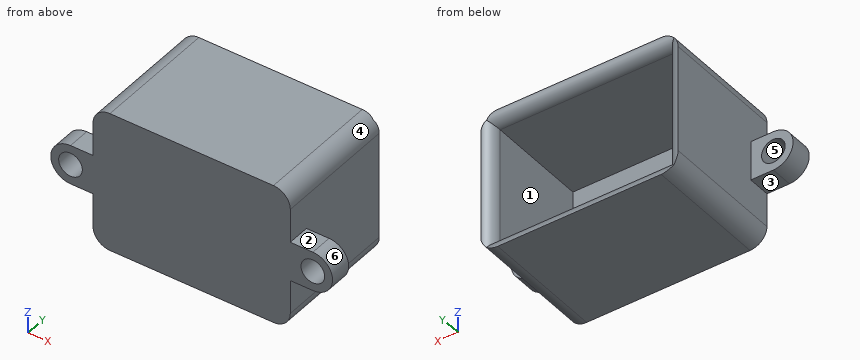
from build123d import *

# Parameters (mm, degrees)
SKETCH2_W           = 35
SKETCH2_H           = 25
SKETCH2_W_2         = 31
SKETCH2_H_2         = 21
BOSS_EXTRUDE1_DEPTH = 20
SKETCH3_W           = 35
SKETCH3_H           = 25
BOSS_EXTRUDE2_DEPTH = 2
SKETCH4_R           = 2.1
BOSS_EXTRUDE3_DEPTH = 4
FILLET1_R           = 3
FILLET2_R           = 2


with BuildPart() as part:
    # Sketch2 → Boss-Extrude1 (new body)
    with BuildSketch(Plane(origin=(0, 0, 0), x_dir=(1, 0, 0), z_dir=(0, 1, 0))):
        Rectangle(SKETCH2_W, SKETCH2_H)
        Rectangle(SKETCH2_W_2, SKETCH2_H_2, mode=Mode.SUBTRACT)
    extrude(amount=BOSS_EXTRUDE1_DEPTH)

    # Sketch3 → Boss-Extrude2 (add)
    with BuildSketch(Plane.XZ):
        Rectangle(SKETCH3_W, SKETCH3_H)
    extrude(amount=BOSS_EXTRUDE2_DEPTH)

    # Sketch4 → Boss-Extrude3 (add)
    # profile 1 of 2: a face of its own
    with BuildSketch(Plane.XZ.offset(2)):
        with BuildLine():
            Line((-21.5, 3.5), (-17.5, 3.5))
            Line((-17.5, 3.5), (-17.5, -3.5))
            Line((-17.5, -3.5), (-21.5, -3.5))
            ThreePointArc((-21.5, -3.5), (-25, 0), (-21.5, 3.5))
        make_face()
        with Locations(Location((-21.5, 0, 0), (0, 0, 270))):
            Circle(SKETCH4_R, mode=Mode.SUBTRACT)
    # profile 2 of 2: a face of its own
    with BuildSketch(Plane.XZ.offset(2)):
        with BuildLine():
            Line((17.5, 3.5), (17.5, -3.5))
            Line((17.5, -3.5), (21.5, -3.5))
            ThreePointArc((21.5, -3.5), (25, 0), (21.5, 3.5))
            Line((21.5, 3.5), (17.5, 3.5))
        make_face()
        with Locations(Location((21.5, 0, 0), (0, 0, 90))):
            Circle(SKETCH4_R, mode=Mode.SUBTRACT)
    extrude(amount=-BOSS_EXTRUDE3_DEPTH)

    # Fillet1
    fillet1_edges = [part.edges().sort_by_distance(p)[0] for p in [
        (17.5, 9, 12.5),
        (-17.5, 9, 12.5),
        (-17.5, 9, -12.5),
        (17.5, 9, -12.5),
    ]]
    fillet(fillet1_edges, radius=FILLET1_R)

    # Fillet2
    # the kernel refuses this fillet: 2 mm, written as the material it takes off along each edge
    with BuildSketch(Plane(origin=(15.5, 20, -10.5), x_dir=(1, 0, 0), z_dir=(0, 0, 1)), Plane(origin=(-15.5, 20, 10.5), x_dir=(-1, 0, 0), z_dir=(0, 0, -1))) as fillet2_piece_1:
        with BuildLine():
            CenterArc((FILLET2_R, -FILLET2_R), FILLET2_R, 90, 90)
            Line((0, -FILLET2_R), (-FILLET2_R * 0.02, -FILLET2_R))
            Line((-FILLET2_R * 0.02, -FILLET2_R), (-FILLET2_R * 0.02, FILLET2_R * 0.02))
            Line((-FILLET2_R * 0.02, FILLET2_R * 0.02), (FILLET2_R, FILLET2_R * 0.02))
            Line((FILLET2_R, FILLET2_R * 0.02), (FILLET2_R, 0))
        make_face()
    extrude(amount=21, mode=Mode.SUBTRACT)
    with BuildSketch(Plane(origin=(-15.5, 20, -10.5), x_dir=(0, 0, -1), z_dir=(1, 0, 0)), Plane(origin=(15.5, 20, 10.5), x_dir=(0, 0, 1), z_dir=(-1, 0, 0))) as fillet2_piece_2:
        with BuildLine():
            CenterArc((FILLET2_R, -FILLET2_R), FILLET2_R, 90, 90)
            Line((0, -FILLET2_R), (-FILLET2_R * 0.02, -FILLET2_R))
            Line((-FILLET2_R * 0.02, -FILLET2_R), (-FILLET2_R * 0.02, FILLET2_R * 0.02))
            Line((-FILLET2_R * 0.02, FILLET2_R * 0.02), (FILLET2_R, FILLET2_R * 0.02))
            Line((FILLET2_R, FILLET2_R * 0.02), (FILLET2_R, 0))
        make_face()
    extrude(amount=31, mode=Mode.SUBTRACT)
    with BuildSketch(Plane(origin=(15.5, 20, -15.5), x_dir=(1, 0, 0), z_dir=(0, 0, 1))) as fillet2_piece_3a_section:
        with BuildLine():
            CenterArc((FILLET2_R, -FILLET2_R), FILLET2_R, 90, 90)
            Line((0, -FILLET2_R), (-FILLET2_R * 0.02, -FILLET2_R))
            Line((-FILLET2_R * 0.02, -FILLET2_R), (-FILLET2_R * 0.02, FILLET2_R * 0.02))
            Line((-FILLET2_R * 0.02, FILLET2_R * 0.02), (FILLET2_R, FILLET2_R * 0.02))
            Line((FILLET2_R, FILLET2_R * 0.02), (FILLET2_R, 0))
        make_face()
    fillet2_piece_3a = extrude(amount=26, mode=Mode.PRIVATE)
    fillet2_piece_3a = split(fillet2_piece_3a, bisect_by=Plane(origin=(15.952790229, 19.547209771, -10.5), z_dir=(0, 0, -1)), keep=Keep.TOP, mode=Mode.PRIVATE)
    with BuildSketch(Plane(origin=(-15.5, 20, -10.5), x_dir=(0, 0, -1), z_dir=(1, 0, 0))) as fillet2_piece_3b_section:
        with BuildLine():
            CenterArc((FILLET2_R, -FILLET2_R), FILLET2_R, 90, 90)
            Line((0, -FILLET2_R), (-FILLET2_R * 0.02, -FILLET2_R))
            Line((-FILLET2_R * 0.02, -FILLET2_R), (-FILLET2_R * 0.02, FILLET2_R * 0.02))
            Line((-FILLET2_R * 0.02, FILLET2_R * 0.02), (FILLET2_R, FILLET2_R * 0.02))
            Line((FILLET2_R, FILLET2_R * 0.02), (FILLET2_R, 0))
        make_face()
    fillet2_piece_3b = extrude(amount=36, mode=Mode.PRIVATE)
    fillet2_piece_3b = split(fillet2_piece_3b, bisect_by=Plane(origin=(15.5, 19.547209771, -10.952790229), z_dir=(1, 0, 0)), keep=Keep.TOP, mode=Mode.PRIVATE)
    fillet2_piece_3 = fillet2_piece_3a & fillet2_piece_3b
    add(fillet2_piece_3, mode=Mode.SUBTRACT)
    with BuildSketch(Plane(origin=(20.5, 20, 10.5), x_dir=(0, 0, 1), z_dir=(-1, 0, 0))) as fillet2_piece_4a_section:
        with BuildLine():
            CenterArc((FILLET2_R, -FILLET2_R), FILLET2_R, 90, 90)
            Line((0, -FILLET2_R), (-FILLET2_R * 0.02, -FILLET2_R))
            Line((-FILLET2_R * 0.02, -FILLET2_R), (-FILLET2_R * 0.02, FILLET2_R * 0.02))
            Line((-FILLET2_R * 0.02, FILLET2_R * 0.02), (FILLET2_R, FILLET2_R * 0.02))
            Line((FILLET2_R, FILLET2_R * 0.02), (FILLET2_R, 0))
        make_face()
    fillet2_piece_4a = extrude(amount=36, mode=Mode.PRIVATE)
    fillet2_piece_4a = split(fillet2_piece_4a, bisect_by=Plane(origin=(15.5, 19.547209771, 10.952790229), z_dir=(1, 0, 0)), keep=Keep.TOP, mode=Mode.PRIVATE)
    with BuildSketch(Plane(origin=(15.5, 20, -10.5), x_dir=(1, 0, 0), z_dir=(0, 0, 1))) as fillet2_piece_4b_section:
        with BuildLine():
            CenterArc((FILLET2_R, -FILLET2_R), FILLET2_R, 90, 90)
            Line((0, -FILLET2_R), (-FILLET2_R * 0.02, -FILLET2_R))
            Line((-FILLET2_R * 0.02, -FILLET2_R), (-FILLET2_R * 0.02, FILLET2_R * 0.02))
            Line((-FILLET2_R * 0.02, FILLET2_R * 0.02), (FILLET2_R, FILLET2_R * 0.02))
            Line((FILLET2_R, FILLET2_R * 0.02), (FILLET2_R, 0))
        make_face()
    fillet2_piece_4b = extrude(amount=26, mode=Mode.PRIVATE)
    fillet2_piece_4b = split(fillet2_piece_4b, bisect_by=Plane(origin=(15.952790229, 19.547209771, 10.5), z_dir=(0, 0, 1)), keep=Keep.TOP, mode=Mode.PRIVATE)
    fillet2_piece_4 = fillet2_piece_4a & fillet2_piece_4b
    add(fillet2_piece_4, mode=Mode.SUBTRACT)
    with BuildSketch(Plane(origin=(-15.5, 20, 10.5), x_dir=(-1, 0, 0), z_dir=(0, 0, -1))) as fillet2_piece_5a_section:
        with BuildLine():
            CenterArc((FILLET2_R, -FILLET2_R), FILLET2_R, 90, 90)
            Line((0, -FILLET2_R), (-FILLET2_R * 0.02, -FILLET2_R))
            Line((-FILLET2_R * 0.02, -FILLET2_R), (-FILLET2_R * 0.02, FILLET2_R * 0.02))
            Line((-FILLET2_R * 0.02, FILLET2_R * 0.02), (FILLET2_R, FILLET2_R * 0.02))
            Line((FILLET2_R, FILLET2_R * 0.02), (FILLET2_R, 0))
        make_face()
    fillet2_piece_5a = extrude(amount=26, mode=Mode.PRIVATE)
    fillet2_piece_5a = split(fillet2_piece_5a, bisect_by=Plane(origin=(-15.952790229, 19.547209771, -10.5), z_dir=(0, 0, -1)), keep=Keep.TOP, mode=Mode.PRIVATE)
    with BuildSketch(Plane(origin=(-20.5, 20, -10.5), x_dir=(0, 0, -1), z_dir=(1, 0, 0))) as fillet2_piece_5b_section:
        with BuildLine():
            CenterArc((FILLET2_R, -FILLET2_R), FILLET2_R, 90, 90)
            Line((0, -FILLET2_R), (-FILLET2_R * 0.02, -FILLET2_R))
            Line((-FILLET2_R * 0.02, -FILLET2_R), (-FILLET2_R * 0.02, FILLET2_R * 0.02))
            Line((-FILLET2_R * 0.02, FILLET2_R * 0.02), (FILLET2_R, FILLET2_R * 0.02))
            Line((FILLET2_R, FILLET2_R * 0.02), (FILLET2_R, 0))
        make_face()
    fillet2_piece_5b = extrude(amount=36, mode=Mode.PRIVATE)
    fillet2_piece_5b = split(fillet2_piece_5b, bisect_by=Plane(origin=(-15.5, 19.547209771, -10.952790229), z_dir=(-1, 0, 0)), keep=Keep.TOP, mode=Mode.PRIVATE)
    fillet2_piece_5 = fillet2_piece_5a & fillet2_piece_5b
    add(fillet2_piece_5, mode=Mode.SUBTRACT)
    with BuildSketch(Plane(origin=(-15.5, 20, 15.5), x_dir=(-1, 0, 0), z_dir=(0, 0, -1))) as fillet2_piece_6a_section:
        with BuildLine():
            CenterArc((FILLET2_R, -FILLET2_R), FILLET2_R, 90, 90)
            Line((0, -FILLET2_R), (-FILLET2_R * 0.02, -FILLET2_R))
            Line((-FILLET2_R * 0.02, -FILLET2_R), (-FILLET2_R * 0.02, FILLET2_R * 0.02))
            Line((-FILLET2_R * 0.02, FILLET2_R * 0.02), (FILLET2_R, FILLET2_R * 0.02))
            Line((FILLET2_R, FILLET2_R * 0.02), (FILLET2_R, 0))
        make_face()
    fillet2_piece_6a = extrude(amount=26, mode=Mode.PRIVATE)
    fillet2_piece_6a = split(fillet2_piece_6a, bisect_by=Plane(origin=(-15.952790229, 19.547209771, 10.5), z_dir=(0, 0, 1)), keep=Keep.TOP, mode=Mode.PRIVATE)
    with BuildSketch(Plane(origin=(15.5, 20, 10.5), x_dir=(0, 0, 1), z_dir=(-1, 0, 0))) as fillet2_piece_6b_section:
        with BuildLine():
            CenterArc((FILLET2_R, -FILLET2_R), FILLET2_R, 90, 90)
            Line((0, -FILLET2_R), (-FILLET2_R * 0.02, -FILLET2_R))
            Line((-FILLET2_R * 0.02, -FILLET2_R), (-FILLET2_R * 0.02, FILLET2_R * 0.02))
            Line((-FILLET2_R * 0.02, FILLET2_R * 0.02), (FILLET2_R, FILLET2_R * 0.02))
            Line((FILLET2_R, FILLET2_R * 0.02), (FILLET2_R, 0))
        make_face()
    fillet2_piece_6b = extrude(amount=36, mode=Mode.PRIVATE)
    fillet2_piece_6b = split(fillet2_piece_6b, bisect_by=Plane(origin=(-15.5, 19.547209771, 10.952790229), z_dir=(-1, 0, 0)), keep=Keep.TOP, mode=Mode.PRIVATE)
    fillet2_piece_6 = fillet2_piece_6a & fillet2_piece_6b
    add(fillet2_piece_6, mode=Mode.SUBTRACT)


solid = part.part
Could you check a few things on this model? Use its own coordinates, in mm. Face numbers are marked on the shaded views. A direction names the side the tool comes from. Give positions to 0.01 mm unless a question says otherwise; leave off trailing zeros. Order: outer loops, then holes, each group sorted by start corner. A loop starts at its lowest first (then second) coordinate and runs counter-clockwise, first axis right, second up.
1. I need wall thicknesses on L1, parallel to X at y = 0.25, z = 0; L2, parallel to X at y = -0.65, z = 0; L3, parallel to X at y = 3, z = 1. Which ranges of each line are inside material? Lowest first, please.
2. For the marked faces 1, 2 and 3, which set-ups out of +Z, -Z, +X, -X, +Y, -Y let a thin tool reach every point of the face, with its end or its side?
3. Will these pins go through, and if not, where does the flat tip stop? P1, Ø2, axis at x = -19, y = 0, coming from the -Z side; P2, Ø7.5, axis at x = -23, z = 1.5, coming from the +Y side; P3, Ø1, axis at y = 10.5, z = -7, coming from the -X side.
4. Suppose I cut it at A-A (z = 0). List the corners of the cut face in (x, y) for me.
5. Suppose I cut it at C-C (y = 7.25). List the corners of the cut face in (x, z) for me.
6. We'd pull the mould along Z, two halves only. Please class the marked faces 4, 5 and 6: pulls with the +Z half, pulls with the -Z half, needs draft (parallel to the pull), parting line crosses it, or undercut.
7. Suppose I cut it at B-B (z = 7.25). List the corners of the cut face in (x, y) for me, plus the area to 3 significant figures.
8. Suppose I cut it at D-D (x = -1). List the corners of the cut face in (y, z) for me, plus the area to 3 significant figures.
Solved:
1. L1: x = -25 to -23.6, -19.4 to -15.5, 15.5 to 19.4, 23.6 to 25
1. L2: x = -25 to -23.6, -19.4 to 19.4, 23.6 to 25
1. L3: x = -17.5 to -15.5, 15.5 to 17.5
2. face 1: +Y
2. face 2: +Z, +X, +Y, -Y
2. face 3: -Z, -X, +Y, -Y
3. P1: stops at z = -3.5
3. P2: stops at y = 2
3. P3: stops at x = -17.5
4. outline: (-25, -2) - (-23.6, -2) - (-23.6, 2) - (-25, 2) - close; (-19.4, -2) - (19.4, -2) - (19.4, 2) - (17.5, 2) - (17.5, 20) arc R2 ccw to (15.5, 18) - (15.5, 0) - (-15.5, 0) - (-15.5, 18) arc R2 ccw to (-17.5, 20) - (-17.5, 2) - (-19.4, 2) - close; (23.6, -2) - (25, -2) - (25, 2) - (23.6, 2) - close
5. outline: (-17.5, -9.5) arc R3 ccw to (-14.5, -12.5) - (14.5, -12.5) arc R3 ccw to (17.5, -9.5) - (17.5, 9.5) arc R3 ccw to (14.5, 12.5) - (-14.5, 12.5) arc R3 ccw to (-17.5, 9.5) - close; hole (-15.5, -10.5) - (15.5, -10.5) - (15.5, 10.5) - (-15.5, 10.5) - close
6. face 4: pulls with the +Z half
6. face 5: undercut
6. face 6: parting line crosses it
7. outline: (-17.5, -2) - (17.5, -2) - (17.5, 20) arc R2 ccw to (15.5, 18) - (15.5, 0) - (-15.5, 0) - (-15.5, 18) arc R2 ccw to (-17.5, 20) - close
7. area: 148 mm2
8. outline: (-2, -12.5) - (20, -12.5) arc R2 ccw to (18, -10.5) - (0, -10.5) - (0, 10.5) - (18, 10.5) arc R2 ccw to (20, 12.5) - (-2, 12.5) - close
8. area: 128 mm2
